Verification items for the finished model (mm, model axes). A direction names the side the tool comes from. Coordinates: 2 decimals unless noted, no trailing zeros. Order: outer loops, then holes, each group sorted by start corner. A loop starts at its lowest first (then second) coordinate and runs counter-clockwise, first axis right, second up.
Q1. Draft check along Y on faces 3 (the flat face through (19.75, -41.52, 4.44)), 4 (the cylindrical face through (37.753, 0.121, 4.437)), 5 (the flat face through (35.174, 29.611, 4.437)). Enter one of: pulls with the +Y half, pulls with the -Y half, needs draft (parallel to the pull), parting line crosses it, or undercut.
Q2. Depth check by flat-ended pin: P1, Ø1.5, axis at y = -14.5, z = 2.5, coming from the +X side; P2, Ø5, axis at x = -19, z = 5.5, coming from the -Y side; P3, Ø4.5, axis at x = 14.845, y = 14.845, coming from the -Z side; P4, Ø4.5, axis at x = 40.5, y = 0, coming from the -Z side. Enter the tip coordinate at first touch or a pass-through.
Q3. Cross-section at B-B, the plane z = 7.5. Count the separate pieces of the cut face and the enclosed holes in it, and give its area (3 significant figures).
Q4. Thickness scan on line 1 (Y direction, x = 13.5, z = 2.5); line 2 (Y direction, x = -6, z = 2); line 3 (Y direction, x = 22, z = 5.25). Record the ranges inside material, lowest first.
Q5. Set-up check for faces 1 (the flat face through (14.6, -43.6, 4.4)), 2 (the flat face through (12, 0, 4)): record each of +Z, -Z, +X, -X, +Y, -Y from which the full face is reachable in a straight line by a thin tool's end or side.
Q6. Cross-section at A-A, the plane y = 1.5. Record the boundary of the cut face in (x, z).
from build123d import *

# Parameters (mm, degrees)
SKETCH_1_R        = 3.75
SKETCH_1_R_2      = 2.75
EXTRUDE_422_DEPTH = 4
EXTRUDE_START     = 4
SKETCH_2_R        = 1.7
SKETCH_2_R_2      = 2.75
EXTRUDE_698_DEPTH = 5


with BuildPart() as part:
    # 草图1 → Extrude 422 (new body)
    with BuildSketch(Plane.XY):
        Polygon((-44.899888641, -10), (-44.2082264, -12.713485699), (-43.352738806, -15.379858192), (-42.336596099, -17.989236526), (-41.163563864, -20.531950955), (-39.837989085, -22.998578775), (-38.364784033, -25.379979238), (-36.74940806, -27.667327432), (-34.997847373, -29.852146979), (-33.116592846, -31.926341448), (-31.112615968, -33.882224361), (-28.993343009, -35.712547671), (-26.7666275, -37.410528629), (-24.440721127, -38.969874914), (-22.024243155, -40.384807953), (-19.526148488, -41.650084336), (-16.955694479, -42.761015244), (-14.322406631, -43.713483827), (-11.636043292, -44.503960459), (-8.906559497, -45.129515818), (-6.144070075, -45.587831742), (-3.358812166, -45.87720982), (-0.561107284, -45.996577684), (2.238676931, -45.945492985), (5.030165132, -45.72414503), (7.803012717, -45.333354084), (10.546944161, -44.774568327), (13.251791096, -44.049858487), (15.907529991, -43.161910171), (18.504319299, -42.114013906), (21.032535927, -40.910052952), (23.482810893, -39.554488905), (25.846064052, -38.052345171), (28.11353774, -36.409188342), (30.276829231, -34.631107573), (32.327921871, -32.724692016), (34.25921479, -30.697006401), (36.063551069, -28.555564857), (37.734244259, -26.308303066), (39.265103162, -23.963548854), (40.650454772, -21.529991333), (41.885165301, -19.016648698), (42.9646592, -16.432834808), (43.884936117, -13.788124675), (44.64258572, -11.092318975), (45.234800338, -8.355407734), (45.659385361, -5.587533306), (45.914767377, -2.798952785), (46, 0), (45.914767377, 2.798952785), (45.659385361, 5.587533306), (45.234800338, 8.355407734), (44.64258572, 11.092318975), (43.884936117, 13.788124675), (42.9646592, 16.432834808), (41.885165301, 19.016648698), (40.650454772, 21.529991333), (39.265103162, 23.963548854), (37.734244259, 26.308303066), (36.063551069, 28.555564857), (34.25921479, 30.697006401), (32.327921871, 32.724692016), (30.276829231, 34.631107573), (28.11353774, 36.409188342), (25.846064052, 38.052345171), (23.482810893, 39.554488905), (21.032535927, 40.910052952), (18.504319299, 42.114013906), (15.907529991, 43.161910171), (13.251791096, 44.049858487), (10.546944161, 44.774568327), (7.803012717, 45.333354084), (5.030165132, 45.72414503), (2.238676931, 45.945492985), (-0.561107284, 45.996577684), (-3.358812166, 45.87720982), (-6.144070075, 45.587831742), (-8.906559497, 45.129515818), (-11.636043292, 44.503960459), (-14.322406631, 43.713483827), (-16.955694479, 42.761015244), (-19.526148488, 41.650084336), (-22.024243155, 40.384807953), (-24.440721127, 38.969874914), (-26.7666275, 37.410528629), (-28.993343009, 35.712547671), (-31.112615968, 33.882224361), (-33.116592846, 31.926341448), (-34.997847373, 29.852146979), (-36.74940806, 27.667327432), (-38.364784033, 25.379979238), (-39.837989085, 22.998578775), (-41.163563864, 20.531950955), (-42.336596099, 17.989236526), (-43.352738806, 15.379858192), (-44.2082264, 12.713485699), (-44.899888641, 10), (12, 10), (12, -10), align=None)
        with Locations((-14.845, -14.845)):
            Circle(SKETCH_1_R, mode=Mode.SUBTRACT)
        with Locations((-14.845, 14.845)):
            Circle(SKETCH_1_R, mode=Mode.SUBTRACT)
        with Locations((14.845, -14.845)):
            Circle(SKETCH_1_R, mode=Mode.SUBTRACT)
        with Locations((14.845, 14.845)):
            Circle(SKETCH_1_R, mode=Mode.SUBTRACT)
        with Locations((0, -40.5)):
            Circle(SKETCH_1_R_2, mode=Mode.SUBTRACT)
        with Locations((0, 40.5)):
            Circle(SKETCH_1_R_2, mode=Mode.SUBTRACT)
        with Locations((40.5, 0)):
            Circle(SKETCH_1_R_2, mode=Mode.SUBTRACT)
    extrude(amount=EXTRUDE_422_DEPTH)

    # 草图2 → Extrude 698 (add)
    with BuildSketch(Plane.XY.offset(EXTRUDE_START)):
        Polygon((-44.899888641, -10), (-44.2082264, -12.713485699), (-43.352738806, -15.379858192), (-42.336596099, -17.989236526), (-41.163563864, -20.531950955), (-39.837989085, -22.998578775), (-38.364784033, -25.379979238), (-36.74940806, -27.667327432), (-34.997847373, -29.852146979), (-33.116592846, -31.926341448), (-31.112615968, -33.882224361), (-28.993343009, -35.712547671), (-26.7666275, -37.410528629), (-24.440721127, -38.969874914), (-22.024243155, -40.384807953), (-19.526148488, -41.650084336), (-16.955694479, -42.761015244), (-14.322406631, -43.713483827), (-11.636043292, -44.503960459), (-8.906559497, -45.129515818), (-6.144070075, -45.587831742), (-3.358812166, -45.87720982), (-0.561107284, -45.996577684), (2.238676931, -45.945492985), (5.030165132, -45.72414503), (7.803012717, -45.333354084), (10.546944161, -44.774568327), (13.251791096, -44.049858487), (15.907529991, -43.161910171), (18.504319299, -42.114013906), (21.032535927, -40.910052952), (23.482810893, -39.554488905), (25.846064052, -38.052345171), (28.11353774, -36.409188342), (30.276829231, -34.631107573), (32.327921871, -32.724692016), (34.25921479, -30.697006401), (36.063551069, -28.555564857), (37.734244259, -26.308303066), (39.265103162, -23.963548854), (40.650454772, -21.529991333), (41.885165301, -19.016648698), (42.9646592, -16.432834808), (43.884936117, -13.788124675), (44.64258572, -11.092318975), (45.234800338, -8.355407734), (45.659385361, -5.587533306), (45.914767377, -2.798952785), (46, 0), (45.914767377, 2.798952785), (45.659385361, 5.587533306), (45.234800338, 8.355407734), (44.64258572, 11.092318975), (43.884936117, 13.788124675), (42.9646592, 16.432834808), (41.885165301, 19.016648698), (40.650454772, 21.529991333), (39.265103162, 23.963548854), (37.734244259, 26.308303066), (36.063551069, 28.555564857), (34.25921479, 30.697006401), (32.327921871, 32.724692016), (30.276829231, 34.631107573), (28.11353774, 36.409188342), (25.846064052, 38.052345171), (23.482810893, 39.554488905), (21.032535927, 40.910052952), (18.504319299, 42.114013906), (15.907529991, 43.161910171), (13.251791096, 44.049858487), (10.546944161, 44.774568327), (7.803012717, 45.333354084), (5.030165132, 45.72414503), (2.238676931, 45.945492985), (-0.561107284, 45.996577684), (-3.358812166, 45.87720982), (-6.144070075, 45.587831742), (-8.906559497, 45.129515818), (-11.636043292, 44.503960459), (-14.322406631, 43.713483827), (-16.955694479, 42.761015244), (-19.526148488, 41.650084336), (-22.024243155, 40.384807953), (-24.440721127, 38.969874914), (-26.7666275, 37.410528629), (-28.993343009, 35.712547671), (-31.112615968, 33.882224361), (-33.116592846, 31.926341448), (-34.997847373, 29.852146979), (-36.74940806, 27.667327432), (-38.364784033, 25.379979238), (-39.837989085, 22.998578775), (-41.163563864, 20.531950955), (-42.336596099, 17.989236526), (-43.352738806, 15.379858192), (-44.2082264, 12.713485699), (-44.899888641, 10), (12, 10), (12, -10), align=None)
        with Locations((-14.845, -14.845)):
            Circle(SKETCH_2_R, mode=Mode.SUBTRACT)
        with Locations((-14.845, 14.845)):
            Circle(SKETCH_2_R, mode=Mode.SUBTRACT)
        with Locations((14.845, -14.845)):
            Circle(SKETCH_2_R, mode=Mode.SUBTRACT)
        with Locations((14.845, 14.845)):
            Circle(SKETCH_2_R, mode=Mode.SUBTRACT)
        with Locations((0, -40.5)):
            Circle(SKETCH_2_R_2, mode=Mode.SUBTRACT)
        with Locations((0, 40.5)):
            Circle(SKETCH_2_R_2, mode=Mode.SUBTRACT)
        with Locations((40.5, 0)):
            Circle(SKETCH_2_R_2, mode=Mode.SUBTRACT)
    extrude(amount=EXTRUDE_698_DEPTH)


solid = part.part
Check values:
1. face 3: pulls with the -Y half
1. face 4: undercut
1. face 5: pulls with the +Y half
2. P1: stops at x = 43.9
2. P2: stops at y = -42.93
2. P3: stops at z = 4
2. P4: passes through
3. separate pieces: 1
3. enclosed holes: 7
3. area: 5,380 mm2
4. line 1: y = -43.97 to -18.35, -11.34 to 11.34, 18.35 to 43.97
4. line 2: y = -45.6 to -10, 10 to 45.6
4. line 3: y = -40.37 to 40.37
5. face 1: +Z, -Z, +X, -Y
5. face 2: +Z, -Z, -X
6. outline: (12, 0) - (38.2, 0) - (38.2, 9) - (12, 9) - close; (42.8, 0) - (45.95, 0) - (45.95, 9) - (42.8, 9) - close
